For this review, take the finished solid that the model builds, in its own axes (mm). A direction names the side the tool comes from. Round coordinates to 2 decimals unless told otherwise and drop trailing zeros. Write each loop counter-clockwise with the first axis right and the second up, starting at its lowest first coordinate (ties: lowest second). Pieces come first, ordered by that corner, then holes. Notation, with made-up numbers: M 27,30 L 70,30 A18 ccw 70,54 Z; hole C 3.5,73.5 d6. An arc over 180 degrees is marked long. Use one line per item in the form item = value. Start each with the question number.
Item 1: For P1, Ø5.5, axis at x = -85.075, y = 156.8, coming from the +Z side; P2, Ø8, axis at y = 23, z = 31, coming from the +X side; P3, Ø10, axis at x = -30, y = 72.5, coming from the -Z side, all flat-tipped, find the tip position at first contact; note any pin that passes through.
Item 2: Add section B-B (z = 0). State the section outline as (x, y) points (3 decimals).
Item 3: Add section A-A (x = 0). State the section outline as (y, z) points (3 decimals).
Item 4: For faces 1 (the flat face through (-91, 0, 30)), 2 (the flat face through (-51, 25.4, -81)), list the 3-axis set-ups (+Z, -Z, +X, -X, +Y, -Y) from which the entire face can be reached by the end or side of a thin tool; tool diameter is ignored.
Item 5: Add section D-D (x = -76). State the section outline as (y, z) points.
Item 6: For line 1 (Y direction, x = 0, z = -97) (3 decimals); line 2 (X direction, y = 132.5, z = 21); line 3 (Z direction, x = -19, y = 48), list the stretches that pass through material, from the lowest coordinate up. Write a range as [from, to].
Item 7: Add section C-C (y = 12.7). State the section outline as (x, z) points (3 decimals).
Item 8: Draft analysis for pull direction X (two halves, no side actions). For faces 3 (the cylindrical face through (-22.025, 84.525, 99.184)), 4 (the cylindrical face through (-75.587, 12.522, 57.958)), 5 (the flat face through (-83.3, 171.45, -53.2)), state which applies: released by +X, released by -X, zero draft, split by the parting line, or undercut.
from build123d import *

# Parameters (mm, degrees)
SKETCH1_R               = 101.6
SKETCH1_R_2             = 95.25
BOSS_EXTRUDE1_DEPTH     = 25.4
SKETCH2_R               = 3.175
CUT_EXTRUDE1_DEPTH      = 102.6
CUT_EXTRUDE1_DEPTH_BACK = 102.6
SKETCH5_R               = 101.6
SKETCH5_R_2             = 98.425
BOSS_EXTRUDE2_DEPTH     = 146.05
SKETCH9_R               = 2.1
CUT_EXTRUDE5_DEPTH      = 204.2000001


with BuildPart() as part:
    # Sketch1 → Boss-Extrude1 (new body)
    with BuildSketch(Plane(origin=(0, 0, 0), x_dir=(1, 0, 0), z_dir=(0, 1, 0))):
        Circle(SKETCH1_R)
        Circle(SKETCH1_R_2, mode=Mode.SUBTRACT)
    extrude(amount=BOSS_EXTRUDE1_DEPTH)

    # Sketch2 → Cut-Extrude1 (cut, two sides)
    with BuildSketch(Plane.XY) as cut_extrude1_sk:
        with Locations((0, 12.7)):
            Circle(SKETCH2_R)
    extrude(amount=CUT_EXTRUDE1_DEPTH, mode=Mode.SUBTRACT)
    extrude(cut_extrude1_sk.sketch, amount=-CUT_EXTRUDE1_DEPTH_BACK, mode=Mode.SUBTRACT)

    # Sketch5 → Boss-Extrude2 (add)
    with BuildSketch(Plane(origin=(0, 25.4, 0), x_dir=(1, 0, 0), z_dir=(0, 1, 0))):
        Circle(SKETCH5_R)
        Circle(SKETCH5_R_2, mode=Mode.SUBTRACT)
    extrude(amount=BOSS_EXTRUDE2_DEPTH)

    # Sketch9 → Cut-Extrude5 (cut, through all)
    with BuildSketch(Plane.XY.offset(101.6)):
        with Locations((-85.075, 156.8)):
            Circle(SKETCH9_R)
    extrude(amount=-CUT_EXTRUDE5_DEPTH, mode=Mode.SUBTRACT)


solid = part.part
Calculated:
q1.P1 = 59.54
q1.P2 = 97.95
q1.P3 = -98.48
q2.outline = M -101.6,0 L -95.25,0 L -95.25,25.4 L -98.425,25.4 L -98.425,171.45 L -101.6,171.45 Z; M 95.25,0 L 101.6,0 L 101.6,171.45 L 98.425,171.45 L 98.425,25.4 L 95.25,25.4 Z
q3.outline = M 0,-101.6 L 9.525,-101.6 L 9.525,-95.25 L 0,-95.25 Z; M 0,95.25 L 9.525,95.25 L 9.525,101.6 L 0,101.6 Z; M 15.875,-101.6 L 171.45,-101.6 L 171.45,-98.425 L 25.4,-98.425 L 25.4,-95.25 L 15.875,-95.25 Z; M 15.875,95.25 L 25.4,95.25 L 25.4,98.425 L 171.45,98.425 L 171.45,101.6 L 15.875,101.6 Z
q4.face_1 = +Z, -Z, +X, -X, -Y
q4.face_2 = +Y
q5.outline = M 0,-67.43 L 171.45,-67.43 L 171.45,-62.54 L 25.4,-62.54 L 25.4,-57.42 L 0,-57.42 Z; M 0,57.42 L 25.4,57.42 L 25.4,62.54 L 171.45,62.54 L 171.45,67.43 L 0,67.43 Z
q6.line_1 = [0, 9.525], [15.875, 25.4]
q6.line_2 = [-99.41, -96.16], [96.16, 99.41]
q6.line_3 = [-99.81, -96.57], [96.57, 99.81]
q7.outline = M -3.175,-101.55 L -3.175,-95.197 A95.25 cw -3.175,95.197 L -3.175,101.55 A101.6 ccw Z; M 3.175,-101.55 A101.6 ccw 3.175,101.55 L 3.175,95.197 A95.25 cw 3.175,-95.197 Z
q8.face_3 = split by the parting line
q8.face_4 = undercut
q8.face_5 = zero draft
